Source: three-view drawing plus pictorial views. Frame: mm from the lowest corner of the part. Coordinates: 2 decimals unless noted, no trailing zeros. Loops run counter-clockwise (first coordinate to the right, second up) from the corner with the lowest first, then second, coordinate; pieces in that order, holes last. Notation, with made-up numbers: (87, 1) - (119, 1) arc R24 ccw to (119, 26) - close; hole circle Ø11 at (-15.75, 57.5). An arc over 180 degrees is marked (long way). Return JSON: item names as keys, results as strings.
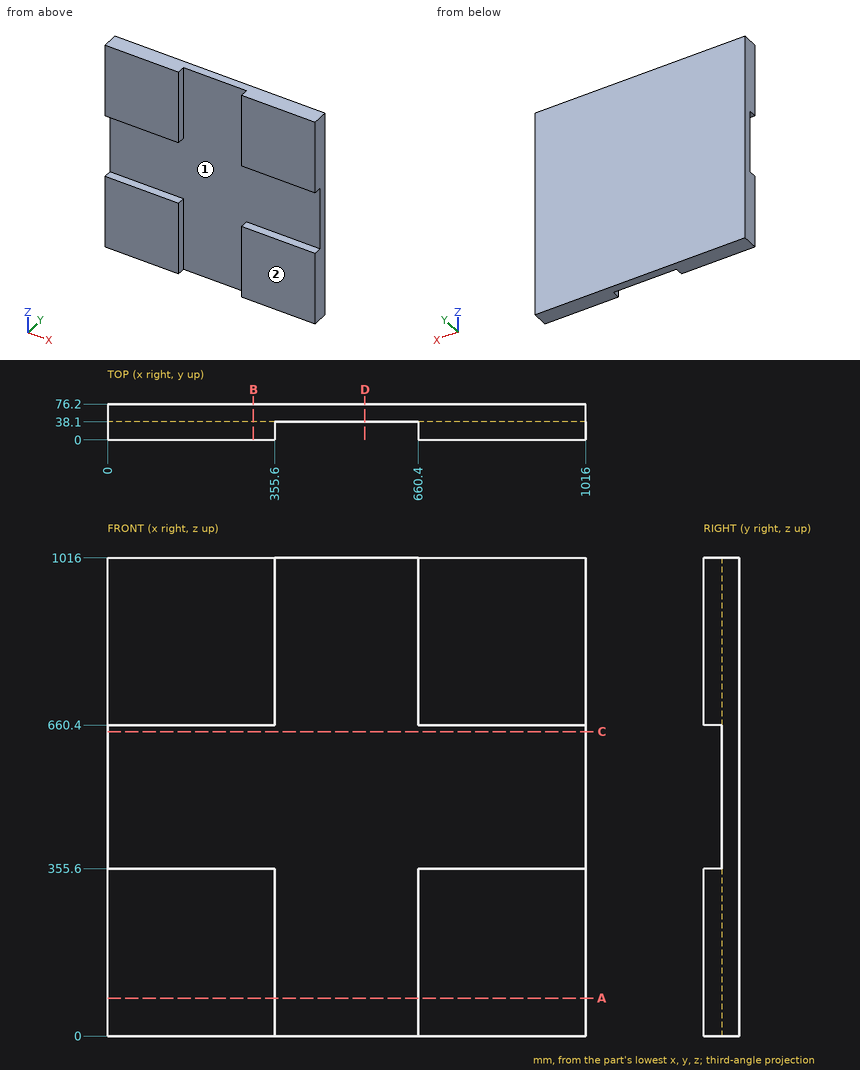
Item 1: Section query A-A, the plane z = 80.5. Return loops of the section in (x, y), and give its area (3 significant figures).
Worked out:
{"outline": "(0, 0) - (355.6, 0) - (355.6, 38.1) - (660.4, 38.1) - (660.4, 0) - (1016, 0) - (1016, 76.2) - (0, 76.2) - close", "area": "65,800 mm^2"}
Item 2: Section query D-D, the plane x = 547. Return loops of the section in (y, z), and give its area (3 significant figures).
Worked out:
{"outline": "(38.1, 0) - (76.2, 0) - (76.2, 1016) - (38.1, 1016) - close", "area": "38,700 mm^2"}
Item 3: Mould query, pull axis X, two halves, no side actions, for the marked faces 1 and 2. Classes: +X half, -X half, draft (parallel to the pull), parting line (faces both ways), or undercut.
Worked out:
{"face 1": "undercut", "face 2": "draft"}
Item 4: Section query B-B, the plane x = 310. Return loops of the section in (y, z), and give its area (3 significant figures).
Worked out:
{"outline": "(0, 0) - (76.2, 0) - (76.2, 1016) - (0, 1016) - (0, 660.4) - (38.1, 660.4) - (38.1, 355.6) - (0, 355.6) - close", "area": "65,800 mm^2"}
Item 5: Section query C-C, the plane z = 647. Return loops of the section in (x, y), and give its area (3 significant figures).
Worked out:
{"outline": "(0, 38.1) - (1016, 38.1) - (1016, 76.2) - (0, 76.2) - close", "area": "38,700 mm^2"}
Item 6: First-contact query: pin 1 Ø5 at (x, z) = (556, 548) entering from -Y. Flat tip, straight axial feed; report the tip coordinate or a pass-through.
Worked out:
{"pin 1": "y = 38.1"}
Item 7: Ray query, probe 1 along X at (y, z) = (28.5, 245.5); probe 2 along Y at (x, z) = (931, 403.5). Return the intervals inside material, ascending. Write a range as from..to.
Worked out:
{"probe 1": "0..355.6, 660.4..1016", "probe 2": "38.1..76.2"}
